Part model, mm, in its own coordinate system. Give positions to 0.01 mm unless a question says otherwise; leave off trailing zeros. Write each loop counter-clockwise with the first axis right and the second up, starting at its lowest first coordinate (ties: lowest second). Pieces come first, ordered by that corner, then holes. Notation, with made-up numbers: M 7.25,37 L 36.25,37 A26 ccw 36.25,75 Z; hole C 49,54.5 d4. An arc over 180 degrees is marked long. Answer as CSV lines item,"result". Start each with the question number.
1) Slice it at A-A, the plane x = -31. Give the cut face in (y, z).
2) Slice it at C-C, the plane z = 0.65. Give the cut face in (x, y), plus the area to 3 significant figures.
3) Wall check: line 1 along Y through (x, z) = (-31, 0.7); line 2 along X through (y, z) = (-30, 0.85); line 3 along Y through (x, z) = (-32.5, 0.9). Give the ranges that are in metal, low to high. Write a range as from..to.
```python
from build123d import *

# Parameters (mm, degrees)
SKETCH_1_W          = 68
SKETCH_1_H          = 68
SKETCH_1_R          = 2.5
SKETCH_1_H_2        = 11
SKETCH_1_W_2        = 11
EXTRUDE_2_DEPTH     = 1
FILLET_1_R          = 3
SKETCH_2_W          = 7.5
SKETCH_2_H          = 68
SKETCH_2_W_2        = 68
SKETCH_2_H_2        = 7.5
CUT_EXTRUDE_1_DEPTH = 2


with BuildPart() as part:
    # ｽｹｯﾁ1 → ﾎﾞｽ - 押し出し2 (new body)
    with BuildSketch(Plane.XY):
        Rectangle(SKETCH_1_W, SKETCH_1_H)
        with Locations((-31, -31)):
            Circle(SKETCH_1_R, mode=Mode.SUBTRACT)
        with Locations((31, -31)):
            Circle(SKETCH_1_R, mode=Mode.SUBTRACT)
        with Locations((-31, 31)):
            Circle(SKETCH_1_R, mode=Mode.SUBTRACT)
        with Locations((31, 31)):
            Circle(SKETCH_1_R, mode=Mode.SUBTRACT)
        with Locations((0, 39.5)):
            Rectangle(SKETCH_1_W, SKETCH_1_H_2)
        with Locations((-39.5, 0)):
            Rectangle(SKETCH_1_W_2, SKETCH_1_H)
        with Locations((39.5, 0)):
            Rectangle(SKETCH_1_W_2, SKETCH_1_H)
        with Locations((0, -39.5)):
            Rectangle(SKETCH_1_W, SKETCH_1_H_2)
    extrude(amount=EXTRUDE_2_DEPTH)

    # ﾌｨﾚｯﾄ1
    fillet_1_edges = [part.edges().sort_by_distance(p)[0] for p in [
        (-34, -34, 0.5),
        (-34, 34, 0.5),
        (34, 34, 0.5),
        (34, -34, 0.5),
    ]]
    fillet(fillet_1_edges, radius=FILLET_1_R)

    # ｽｹｯﾁ2 → ｶｯﾄ - 押し出し1 (cut, through all)
    with BuildSketch(Plane.XY.offset(1)):
        with Locations((-41.25, 0)):
            Rectangle(SKETCH_2_W, SKETCH_2_H)
        with Locations((0, 41.25)):
            Rectangle(SKETCH_2_W_2, SKETCH_2_H_2)
        with Locations((41.25, 0)):
            Rectangle(SKETCH_2_W, SKETCH_2_H)
        with Locations((0, -41.25)):
            Rectangle(SKETCH_2_W_2, SKETCH_2_H_2)
    extrude(amount=-CUT_EXTRUDE_1_DEPTH, mode=Mode.SUBTRACT)


solid = part.part
```
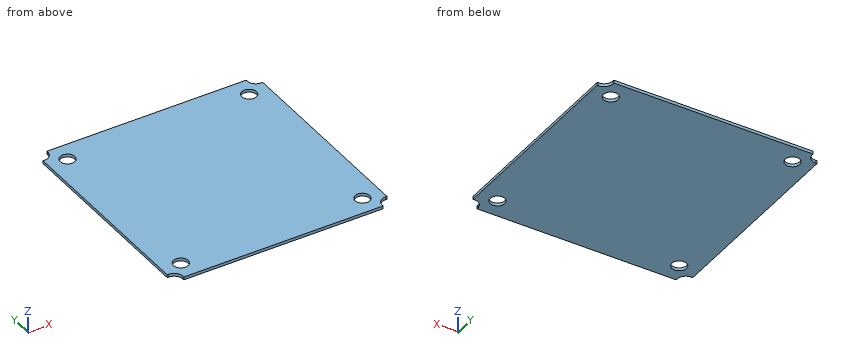
Found:
1,outline,"M -37.5,0 L -33.5,0 L -33.5,1 L -37.5,1 Z; M -28.5,0 L 28.5,0 L 28.5,1 L -28.5,1 Z; M 33.5,0 L 37.5,0 L 37.5,1 L 33.5,1 Z"
2,outline,"M -37.5,-34 L -37,-34 A3 cw -34,-37 L -34,-37.5 L 34,-37.5 L 34,-37 A3 cw 37,-34 L 37.5,-34 L 37.5,34 L 37,34 A3 cw 34,37 L 34,37.5 L -34,37.5 L -34,37 A3 cw -37,34 L -37.5,34 Z; hole C -31,-31 d5; hole C -31,31 d5; hole C 31,-31 d5; hole C 31,31 d5"
2,area,"5,510 mm²"
3,line 1,"-37.5..-33.5, -28.5..28.5, 33.5..37.5"
3,line 2,"-37.5..-33.29, -28.71..28.71, 33.29..37.5"
3,line 3,"-37.5..-33, -29..29, 33..37.5"
